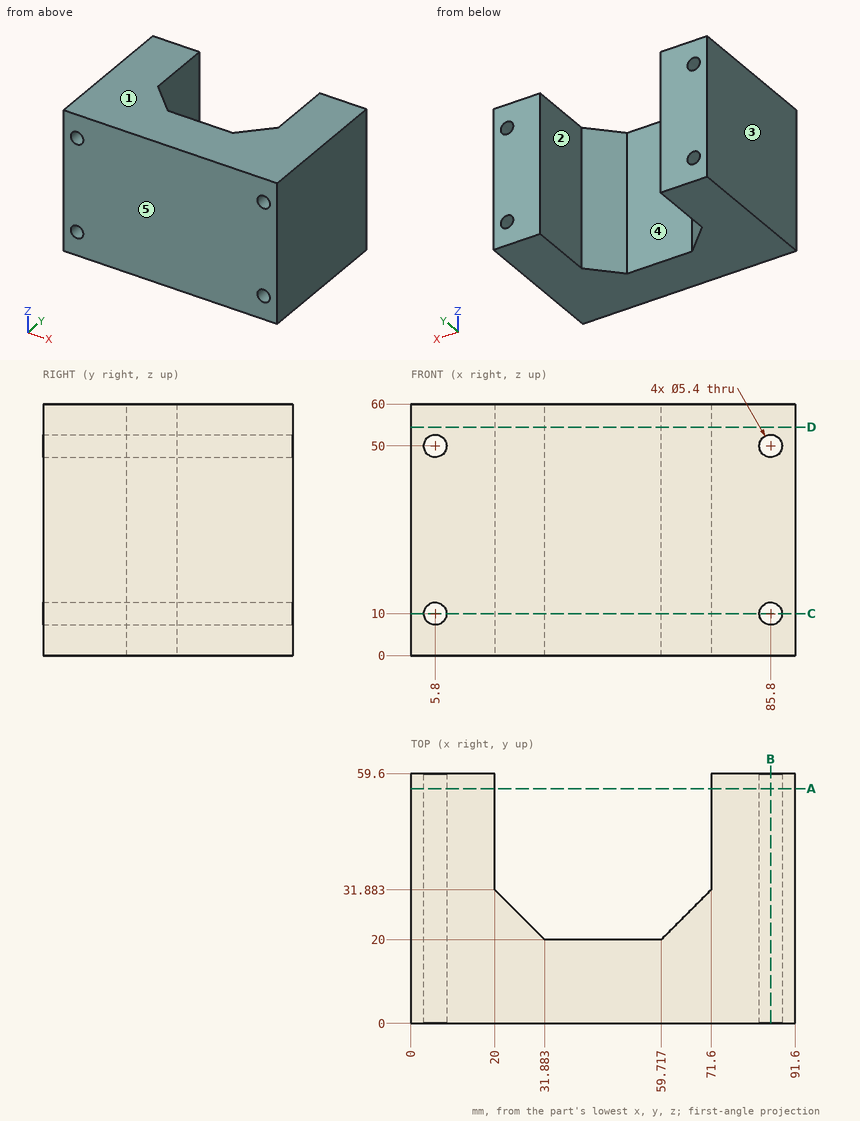
Study the drawing (mm; zero at the part's minimum x, y, z) and answer. A direction names the side the tool comes from. Round coordinates to 2 decimals unless told otherwise and drop trailing zeros. Order: outer loops, then holes, each group sorted by start corner. A loop starts at its lowest first (then second) coordinate and runs counter-clockwise, first axis right, second up. Notation, with made-up numbers: (-18, 25) -> (-1, 25) arc R29 cw to (-1, 62) -> close; hole circle Ø4 at (75.25, 31.5). An arc over 180 degrees is marked (long way). Write each question's results on one line, items separated by ' | '. Start each with the question number.
Q1. The mould has two halves that part along X. Classify the marked faces 3, 4 and 5: pulls with the +X half, pulls with the -X half, needs draft (parallel to the pull), parting line crosses it, or undercut.
Q2. Find section C-C (z = 10). Determine the outline of the cut face in (x, y).
Q3. Find section A-A (y = 56). Determine the outline of the cut face in (x, z), then the cut area to 3 significant figures.
Q4. Straight lines are drawn through the part: probe 1 along Z at (x, y) = (85.8, 18); probe 2 along X at (y, z) = (19, 10); probe 3 along X at (y, z) = (33, 50). For each, find the intervals that lie inside material, in ascending order. Write a range as from..to.
Q5. This flat-tipped pin is pushed along its axis until it touches: pin 1 (2 mm diameter, centred on x = 64, z = 30.5, fed in from +Y). Where does it stop, or does it pass through?
Q6. Find section D-D (z = 54.5). Determine the outline of the cut face in (x, y).
Q7. Which of the six approach directions +Z, -Z, +X, -X, +Y, -Y give full straight-line access (tool end or side, diameter ignored) to the marked faces 1 and 2?
Q8. Find section B-B (x = 85.8). Determine the outline of the cut face in (y, z).
Worked answers:
1) face 3: pulls with the -X half | face 4: undercut | face 5: needs draft
2) outline: (0, 0) -> (3.1, 0) -> (3.1, 59.6) -> (0, 59.6) -> close; (8.5, 0) -> (83.1, 0) -> (83.1, 59.6) -> (71.6, 59.6) -> (71.6, 31.88) -> (59.72, 20) -> (31.88, 20) -> (20, 31.88) -> (20, 59.6) -> (8.5, 59.6) -> close; (88.5, 0) -> (91.6, 0) -> (91.6, 59.6) -> (88.5, 59.6) -> close
3) outline: (0, 0) -> (20, 0) -> (20, 60) -> (0, 60) -> close; (71.6, 0) -> (91.6, 0) -> (91.6, 60) -> (71.6, 60) -> close; hole circle Ø5.4 at (5.8, 10); hole circle Ø5.4 at (5.8, 50); hole circle Ø5.4 at (85.8, 10); hole circle Ø5.4 at (85.8, 50) | area: 2,310 mm2
4) probe 1: z = 0..7.3, 12.7..47.3, 52.7..60 | probe 2: x = 0..3.1, 8.5..83.1, 88.5..91.6 | probe 3: x = 0..3.1, 8.5..20, 71.6..83.1, 88.5..91.6
5) pin 1: stops at y = 25.28
6) outline: (0, 0) -> (91.6, 0) -> (91.6, 59.6) -> (71.6, 59.6) -> (71.6, 31.88) -> (59.72, 20) -> (31.88, 20) -> (20, 31.88) -> (20, 59.6) -> (0, 59.6) -> close
7) face 1: +Z, +X, -X, +Y, -Y | face 2: +Z, -Z, +Y
8) outline: (0, 0) -> (59.6, 0) -> (59.6, 7.3) -> (0, 7.3) -> close; (0, 12.7) -> (59.6, 12.7) -> (59.6, 47.3) -> (0, 47.3) -> close; (0, 52.7) -> (59.6, 52.7) -> (59.6, 60) -> (0, 60) -> close
